Check sheet for the modelled part. Datum: model origin and axes. Units: mm. Face numbers are marked on the shaded views. A direction names the side the tool comes from. Give positions to 0.01 mm unless a question says otherwise; leave off trailing zeros. Order: outer loops, then holes, each group sorted by start corner. A loop starts at its lowest first (then second) coordinate and runs counter-clockwise, first axis right, second up.
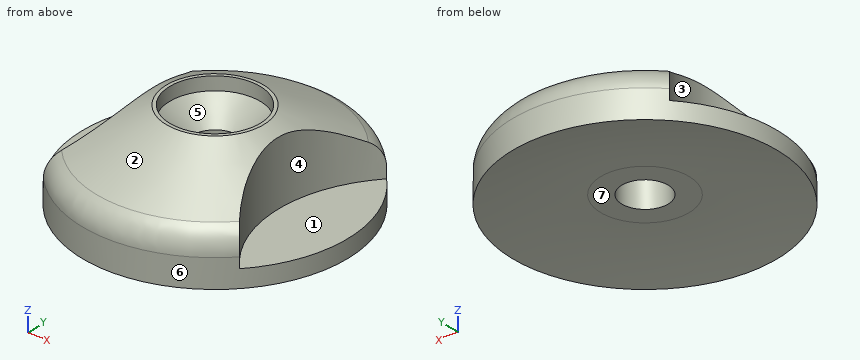
```python
from build123d import *

# Parameters (mm, degrees)
F2_R     = 15
F3_DEPTH = 8


with BuildPart() as f1:
    # F0 (on Front) → F1 (revolve)
    with BuildSketch(Plane.XZ):
        with BuildLine():
            Line((-2.625, 0), (-2.625, 5))
            Line((-2.625, 5), (-5.125, 7.5))
            Line((-5.125, 7.5), (-5.125, 9))
            Line((-5.125, 9), (-5.505, 9))
            Line((-5.505, 9), (-13.402239, 4.843558))
            ThreePointArc((-13.402239, 4.843558), (-14.57324, 3.739333), (-15.005, 2.188804))
            Line((-15.005, 2.188804), (-15.005, -1))
            ThreePointArc((-15.005, -1), (-10.029938, -0.250622), (-5.005, 0))
            Line((-5.005, 0), (-2.625, 0))
        make_face()
    revolve(axis=Axis((0, 0, 10.827172), (0, 0, 1)))

    # F2 (on face) → F3 (cut)
    with BuildSketch(Plane.XY.offset(9)):
        with Locations((-22, 0)):
            Circle(F2_R)
        with Locations((22, 0)):
            Circle(F2_R)
    extrude(amount=-F3_DEPTH, mode=Mode.SUBTRACT)


solid = f1.part
```
(1) Sectioned sample at A-A (z = 1.75). Enter the section's corners in (x, y) (3 decimals), plus the area to 3 significant figures.
(2) Release check for a two-part mould opening along X. For the marked faces 4, 5, 6 and 7 record: released by +X, released by -X, zero draft, split by the parting line, or undercut.
(3) Thickness scan on L1, parallel to Y at x = 0, z = 2 (3 decimals); L2, parallel to X at y = 0, z = 2.05 (3 decimals); L3, parallel to X at y = 0, z = 8.4 (3 decimals). Record the ranges inside material, lowest first.
(4) Tool access check on the marked faces 1, 2 and 3. Record the directions out of +Z, -Z, +X, -X, +Y, -Y that give a thin tool (end or side, any length) a straight path to the whole face; none if there is none.
(5) Go/stop test with flat-tipped pins: P1, Ø4, axis at x = 12, y = -2, coming from the +Z side; P2, Ø1, axis at x = 2.5, y = 7.5, coming from the +Z side; P3, Ø1.5, axis at x = -4, y = 7.5, coming from the -Z side; P4, Ø4, axis at x = 0, y = 0, coming from the +Z side. Record where each tip stops, or that it passes through.
Values follow:
1. outline: (-11.003, -10.202) arc R15.005 ccw to (11.003, -10.202) arc R15 cw to (11.003, 10.202) arc R15.005 ccw to (-11.003, 10.202) arc R15 cw to start; hole circle Ø5.25 at (0, 0)
1. area: 461 mm2
2. face 4: released by +X
2. face 5: undercut
2. face 6: split by the parting line
2. face 7: undercut
3. L1: y = -15.005 to -2.625, 2.625 to 15.005
3. L2: x = -7 to -2.625, 2.625 to 7
3. L3: x = -6.645 to -5.125, 5.125 to 6.645
4. face 1: +Z, +X
4. face 2: +Z
4. face 3: +Z, -X
5. P1: stops at z = 1
5. P2: stops at z = 8
5. P3: stops at z = -0.18
5. P4: passes through
